Build history of the part. All positions in model axes, mm. A direction names the side the tool comes from. Coordinates: 2 decimals unless noted, no trailing zeros. Order: outer loops, then holes, each group sorted by start corner. A loop starts at its lowest first (then second) coordinate and runs counter-clockwise, first axis right, second up. Notation, with made-up numbers: (9, -15.5) -> (25, -15.5) arc R23 ccw to (25, 11.5) -> close; hole circle Ø10 at (41, 64). An arc over 180 degrees is marked (long way). Write each question's results on one line, items separated by ' | '.
from build123d import *

# Parameters (mm, degrees)
F0_R     = 1
F0_R_2   = 2
F1_DEPTH = 2
F2_START = 17
F2_DEPTH = 3
F3_DEPTH = 20
F5_DEPTH = 3
F8_DEPTH = 3
F9_DEPTH = 3


with BuildPart() as f1:
    # F0 (on Top) → F1 (new body)
    with BuildSketch(Plane.XY):
        with BuildLine():
            Line((0.9289886274, 6.9380818769), (3.7480664897, 5.9120214469))
            ThreePointArc((3.7480664897, 5.9120214469), (2.3941410033, 6.5778483455), (0.9289886274, 6.9380818769))
        make_face()
        with BuildLine():
            Line((6.8373971656, -1.5), (6.8373971656, 1.5))
            ThreePointArc((6.8373971656, 1.5), (5.73406431, 4.0150350545), (3.7480664897, 5.9120214469))
            Line((3.7480664897, 5.9120214469), (0.9289886274, 6.9380818769))
            ThreePointArc((0.9289886274, 6.9380818769), (-7, 0), (0.9289886274, -6.9380818769))
            Line((0.9289886274, -6.9380818769), (3.7480664897, -5.9120214469))
            ThreePointArc((3.7480664897, -5.9120214469), (5.73406431, -4.0150350545), (6.8373971656, -1.5))
        make_face()
        with Locations((0, -4.5)):
            Circle(F0_R, mode=Mode.SUBTRACT)
        with Locations((-4.5, 0)):
            Circle(F0_R, mode=Mode.SUBTRACT)
        Circle(F0_R_2, mode=Mode.SUBTRACT)
        with Locations((0, 4.5)):
            Circle(F0_R, mode=Mode.SUBTRACT)
        with Locations((4.5, 0)):
            Circle(F0_R, mode=Mode.SUBTRACT)
        with BuildLine():
            ThreePointArc((6.8373971656, 1.5), (6.9592305666, 0.7543937436), (7, 0))
            ThreePointArc((7, 0), (6.9592305666, -0.7543937436), (6.8373971656, -1.5))
            Line((6.8373971656, -1.5), (11.8373971656, -1.5))
            Line((11.8373971656, -1.5), (11.8373971656, 1.5))
            Line((11.8373971656, 1.5), (6.8373971656, 1.5))
        make_face()
        with BuildLine():
            ThreePointArc((6.8373971656, -1.5), (6.9592305666, -0.7543937436), (7, 0))
            ThreePointArc((7, 0), (6.9592305666, 0.7543937436), (6.8373971656, 1.5))
            Line((6.8373971656, 1.5), (6.8373971656, -1.5))
        make_face()
        with BuildLine():
            ThreePointArc((0.9289886274, -6.9380818769), (2.3941410033, -6.5778483455), (3.7480664897, -5.9120214469))
            Line((3.7480664897, -5.9120214469), (0.9289886274, -6.9380818769))
        make_face()
        with BuildLine():
            Line((5.4581672064, -10.6104845508), (3.7480664897, -5.9120214469))
            ThreePointArc((3.7480664897, -5.9120214469), (2.3941410033, -6.5778483455), (0.9289886274, -6.9380818769))
            Line((0.9289886274, -6.9380818769), (2.639089344, -11.6365449808))
            Line((2.639089344, -11.6365449808), (5.4581672064, -10.6104845508))
        make_face()
        with BuildLine():
            ThreePointArc((0.9289886274, 6.9380818769), (2.3941410033, 6.5778483455), (3.7480664897, 5.9120214469))
            Line((3.7480664897, 5.9120214469), (5.4581672064, 10.6104845508))
            Line((5.4581672064, 10.6104845508), (2.639089344, 11.6365449808))
            Line((2.639089344, 11.6365449808), (0.9289886274, 6.9380818769))
        make_face()
    extrude(amount=F1_DEPTH)



with BuildPart() as f2:
    # F0 (on Top) → F2 (new body)
    with BuildSketch(Plane.XY.offset(F2_START)):
        with BuildLine():
            Line((28.8373971656, -1.5), (27.3373971656, -1.5))
            ThreePointArc((27.3373971656, -1.5), (22.4271695266, -15.7036731632), (10.7594794279, -25.175720173))
            Line((10.7594794279, -25.175720173), (11.2725096429, -26.5852591042))
            ThreePointArc((11.2725096429, -26.5852591042), (23.6541478842, -16.5628126584), (28.8373971656, -1.5))
        make_face()
        with BuildLine():
            Line((11.2725096429, -26.5852591042), (10.7594794279, -25.175720173))
            ThreePointArc((10.7594794279, -25.175720173), (9.3640048747, -25.727391949), (7.9404015655, -26.201780603))
            Line((7.9404015655, -26.201780603), (8.4534317805, -27.6113195342))
            Line((8.4534317805, -27.6113195342), (11.2725096429, -26.5852591042))
        make_face()
        with BuildLine():
            ThreePointArc((10.7594794279, 25.175720173), (22.4271695266, 15.7036731632), (27.3373971656, 1.5))
            Line((27.3373971656, 1.5), (28.8373971656, 1.5))
            ThreePointArc((28.8373971656, 1.5), (23.6541478842, 16.5628126584), (11.2725096429, 26.5852591042))
            Line((11.2725096429, 26.5852591042), (10.7594794279, 25.175720173))
        make_face()
        with BuildLine():
            ThreePointArc((7.9404015655, 26.201780603), (9.3640048747, 25.727391949), (10.7594794279, 25.175720173))
            Line((10.7594794279, 25.175720173), (11.2725096429, 26.5852591042))
            Line((11.2725096429, 26.5852591042), (8.4534317805, 27.6113195342))
            Line((8.4534317805, 27.6113195342), (7.9404015655, 26.201780603))
        make_face()
        with BuildLine():
            Line((28.8373971656, 1.5), (27.3373971656, 1.5))
            ThreePointArc((27.3373971656, 1.5), (27.3785186559, 0), (27.3373971656, -1.5))
            Line((27.3373971656, -1.5), (28.8373971656, -1.5))
            Line((28.8373971656, -1.5), (28.8373971656, 1.5))
        make_face()
    extrude(amount=F2_DEPTH)


with BuildPart() as f1_1:
    add(f1.part)

    add(f2.part)  # F3 merges F2
    # F0 (on Top) → F3 (join)
    with BuildSketch(Plane.XY):
        with BuildLine():
            Line((10.7594794279, -25.175720173), (5.4581672064, -10.6104845508))
            Line((5.4581672064, -10.6104845508), (2.639089344, -11.6365449808))
            Line((2.639089344, -11.6365449808), (7.9404015655, -26.201780603))
            ThreePointArc((7.9404015655, -26.201780603), (9.3640048747, -25.727391949), (10.7594794279, -25.175720173))
        make_face()
        with BuildLine():
            ThreePointArc((7.9404015655, 26.201780603), (9.3640048747, 25.727391949), (10.7594794279, 25.175720173))
            Line((10.7594794279, 25.175720173), (11.2725096429, 26.5852591042))
            Line((11.2725096429, 26.5852591042), (8.4534317805, 27.6113195342))
            Line((8.4534317805, 27.6113195342), (7.9404015655, 26.201780603))
        make_face()
        with BuildLine():
            Line((28.8373971656, 1.5), (27.3373971656, 1.5))
            ThreePointArc((27.3373971656, 1.5), (27.3785186559, 0), (27.3373971656, -1.5))
            Line((27.3373971656, -1.5), (28.8373971656, -1.5))
            Line((28.8373971656, -1.5), (28.8373971656, 1.5))
        make_face()
        with BuildLine():
            Line((11.2725096429, -26.5852591042), (10.7594794279, -25.175720173))
            ThreePointArc((10.7594794279, -25.175720173), (9.3640048747, -25.727391949), (7.9404015655, -26.201780603))
            Line((7.9404015655, -26.201780603), (8.4534317805, -27.6113195342))
            Line((8.4534317805, -27.6113195342), (11.2725096429, -26.5852591042))
        make_face()
        with BuildLine():
            Line((27.3373971656, 1.5), (11.8373971656, 1.5))
            Line((11.8373971656, 1.5), (11.8373971656, -1.5))
            Line((11.8373971656, -1.5), (27.3373971656, -1.5))
            ThreePointArc((27.3373971656, -1.5), (27.3785186559, 0), (27.3373971656, 1.5))
        make_face()
        with BuildLine():
            Line((2.639089344, 11.6365449808), (5.4581672064, 10.6104845508))
            Line((5.4581672064, 10.6104845508), (10.7594794279, 25.175720173))
            ThreePointArc((10.7594794279, 25.175720173), (9.3640048747, 25.727391949), (7.9404015655, 26.201780603))
            Line((7.9404015655, 26.201780603), (2.639089344, 11.6365449808))
        make_face()
    extrude(amount=F3_DEPTH)

    # F4 (on face) → F5 (cut)
    with BuildSketch(Plane(origin=(-1.4095389312, -0.513030215, 0), x_dir=(0.3420201433, -0.9396926208, 0), z_dir=(-0.9396926208, -0.3420201433, 0))):
        Polygon((27.3373971656, 15), (27.3373971656, 20), (11.8373971656, 20), (11.8373971656, 2), align=None)
        Polygon((28.8373971656, 0), (28.8373971656, 13.647751184), (12.5650784462, 0), align=None)
    extrude(amount=-F5_DEPTH, mode=Mode.SUBTRACT)

    # F6 (on face) → F8 (cut)
    with BuildSketch(Plane.XZ.offset(1.5)):
        Polygon((28.8373971656, 0), (28.8373971656, 13.647751184), (12.5650784462, 0), align=None)
        Polygon((27.3373971656, 17), (27.3373971656, 20), (11.8373971656, 20), (11.8373971656, 2), (27.3373971656, 15), align=None)
    extrude(amount=-F8_DEPTH, mode=Mode.SUBTRACT)

    # F7 (on face) → F9 (cut)
    with BuildSketch(Plane(origin=(1.4095389312, -0.513030215, 0), x_dir=(0.3420201433, 0.9396926208, 0), z_dir=(0.9396926208, -0.3420201433, 0))):
        Polygon((27.3373971656, 17), (27.3373971656, 20), (11.8373971656, 20), (11.8373971656, 2), (27.3373971656, 15), align=None)
        Polygon((28.8373971656, 0), (28.8373971656, 13.647751184), (12.5650784462, 0), align=None)
    extrude(amount=-F9_DEPTH, mode=Mode.SUBTRACT)


solid = f1_1.part
Item 1: Pull direction X, two halves, no side cores. Call faces 1 (the flat face through (3, 0, 0)), 2 (the flat face through (20.815, -0.021, 6.919)), 3 (the cylindrical face through (-5.3, -0.6, 1)): released by +X, released by -X, zero draft, split by the parting line, or undercut.
Answer:
face 1: zero draft | face 2: released by +X | face 3: undercut
Item 2: Drill centre lines: line 1 (Y direction, x = -4.5, z = 0.8); line 2 (X direction, y = 14.5, z = 4.5); line 3 (Z direction, x = 24, y = 14). Where is each one in solid material? Low to high. Write a range as from..to.
Answer:
line 1: y = -5.36..-1, 1..5.36 | line 2: x = 3.68..6.87 | line 3: z = 17..20
Item 3: Tool access for faces 4 (the cylindrical face through (-0.13, 5.49, 0.99)), 5 (the cylindrical face through (5.71, -4.05, 0.99)), 6 (the flat face through (27.337, 0, 17)): list every direction of +Z, -Z, +X, -X, +Y, -Y with a clear straight run to the whole face (end or side of a thin tool).
Answer:
face 4: +Z, -Z | face 5: +Z, -Z, +X | face 6: +Z, -X
Item 4: Slice it at C-C, the plane x = -4.5. List the corners of the cut face in (y, z), and give its area (3 significant figures).
Answer:
outline: (-5.36, 0) -> (-1, 0) -> (-1, 2) -> (-5.36, 2) -> close; (1, 0) -> (5.36, 0) -> (5.36, 2) -> (1, 2) -> close | area: 17.4 mm^2
Item 5: Slice it at B-B, the plane z = 17.75. List the corners of the cut face in (x, y), and give its area (3 significant figures).
Answer:
outline: (7.94, -26.2) -> (8.45, -27.61) -> (11.27, -26.59) arc R28.88 ccw to (28.84, -1.5) -> (28.84, 1.5) arc R28.88 ccw to (11.27, 26.59) -> (8.45, 27.61) -> (7.94, 26.2) -> (10.76, 25.18) arc R27.38 cw to (27.34, 1.5) -> (27.34, -1.5) arc R27.38 cw to (10.76, -25.18) -> close | area: 107 mm^2
Item 6: Pin check, flat tips, straight feed: pin 1 (10 mm diameter, centred on x = 6, y = -16, fed in from -Z); pin 2 (3 mm diameter, centred on x = 4.5, y = 0, fed in from +Z); pin 3 (8 mm diameter, centred on y = 1, z = 12, fed in from -X); pin 4 (3 mm diameter, centred on x = 8, z = 6, fed in from -Y). Stop position of each tip, or through.
Answer:
pin 1: stops at z = 0 | pin 2: stops at z = 2 | pin 3: stops at x = 18.99 | pin 4: stops at y = -20.05
Item 7: Slice it at A-A, the plane y = 0. List the corners of the cut face in (x, z), and give its area (3 significant figures).
Answer:
outline: (-7, 0) -> (-5.5, 0) -> (-5.5, 2) -> (-7, 2) -> close; (-3.5, 0) -> (-2, 0) -> (-2, 2) -> (-3.5, 2) -> close; (2, 0) -> (3.5, 0) -> (3.5, 2) -> (2, 2) -> close; (5.5, 0) -> (12.57, 0) -> (28.84, 13.65) -> (28.84, 20) -> (27.34, 20) -> (27.34, 15) -> (11.84, 2) -> (5.5, 2) -> close | area: 72.4 mm^2
Item 8: Slice it at D-D, the plane y = -24. List the corners of the cut face in (x, z), and give its area (3 significant figures).
Answer:
outline: (7.14, 10.42) -> (10.33, 11.34) -> (10.33, 13.95) -> (7.14, 13.03) -> close; (13.18, 17) -> (16.06, 17) -> (16.06, 20) -> (13.18, 20) -> close | area: 17.0 mm^2
